Could you check a few things on this model? Use its own coordinates, in mm. A direction names the side the tool comes from. Coordinates: 2 decimals unless noted, no trailing zeros. Write each loop counter-clockwise with the first axis right and the second up, starting at its lowest first coordinate (ties: lowest second). Pieces come first, ordered by that corner, then holes.
```python
from build123d import *

# Parameters (mm, degrees)
CROQUIS2_W              = 140
CROQUIS2_H              = 140
CROQUIS2_R              = 1.5
CROQUIS2_W_2            = 40
CROQUIS2_H_2            = 5
CROQUIS2_W_3            = 5
CROQUIS2_H_3            = 40
SALIENTE_EXTRUIR1_DEPTH = 5


with BuildPart() as part:
    # Croquis2 → Saliente-Extruir1 (new body)
    with BuildSketch(Plane(origin=(0, 0, 0), x_dir=(1, 0, 0), z_dir=(0, 1, 0))):
        with Locations((70, 70)):
            Rectangle(CROQUIS2_W, CROQUIS2_H)
        with Locations(Location((32.5, 127.5, 0), (0, 0, 270))):
            Circle(CROQUIS2_R, mode=Mode.SUBTRACT)
        with Locations(Location((107.5, 127.5, 0), (0, 0, 90))):
            Circle(CROQUIS2_R, mode=Mode.SUBTRACT)
        with Locations(Location((107.5, 12.5, 0), (0, 0, 270))):
            Circle(CROQUIS2_R, mode=Mode.SUBTRACT)
        with Locations(Location((32.5, 12.5, 0), (0, 0, 90))):
            Circle(CROQUIS2_R, mode=Mode.SUBTRACT)
        with Locations((70, 127.5)):
            Rectangle(CROQUIS2_W_2, CROQUIS2_H_2, mode=Mode.SUBTRACT)
        with Locations((70, 12.5)):
            Rectangle(CROQUIS2_W_2, CROQUIS2_H_2, mode=Mode.SUBTRACT)
        with Locations((127.5, 70)):
            Rectangle(CROQUIS2_W_3, CROQUIS2_H_3, mode=Mode.SUBTRACT)
        with Locations((12.5, 70)):
            Rectangle(CROQUIS2_W_3, CROQUIS2_H_3, mode=Mode.SUBTRACT)
    extrude(amount=SALIENTE_EXTRUIR1_DEPTH)


solid = part.part
```
1. If we mould it in two halves opening along Z, with no side actions, what happens to faces 1 (the face through (15, 2, -70)), 2 (the face through (69, 0, -71))? For each: pulls with the +Z half, pulls with the -Z half, needs draft (parallel to the pull), parting line crosses it, or undercut.
Verdict:
face 1: undercut
face 2: needs draft
2. On a 3-axis mill with a long thin cutter (end or side, diameter ignored), from which of +Z, -Z, +X, -X, +Y, -Y can I reach the whole of each face in a straight line? I mean faces 3 (the face through (127, 2, -50)), 4 (the face through (69, 5, -71)). Say none if no direction works.
Verdict:
face 3: +Y, -Y
face 4: +Z, -Z, +X, -X, +Y
3. I want a section at B-B on y = 3.5. Give the number of separate pieces and of enclosed holes in the cut face, plus the area to 3 significant figures.
Verdict:
separate pieces: 1
enclosed holes: 8
area: 18,800 mm2
4. For pin 1 (2.5 mm diameter, centred on x = 107.5, z = -127.5, fed in from -Y), with a flat end and sliding along its axis, tell me the tip position at first contact or that it passes through.
Verdict:
pin 1: passes through
5. I want a section at A-A on z = -79. Please give me the cut outline in (x, y).
Verdict:
outline: (0, 0) - (10, 0) - (10, 5) - (0, 5) - close; (15, 0) - (125, 0) - (125, 5) - (15, 5) - close; (130, 0) - (140, 0) - (140, 5) - (130, 5) - close
6. Please list where these lines run through material, in increasing order: line 1 along X through (y, z) = (3, -70.5); line 2 along Z through (x, y) = (107.5, 1.3); line 3 along Z through (x, y) = (86, 4.5).
Verdict:
line 1: x = 0 to 10, 15 to 125, 130 to 140
line 2: z = -140 to -129, -126 to -14, -11 to 0
line 3: z = -140 to -130, -125 to -15, -10 to 0
